```python
from build123d import *

# Parameters (mm, degrees)
SKETCH3_W = 15
SKETCH3_H = 18.520312213


with BuildPart() as part:
    # Sketch1 → Revolve1 (revolve)
    with BuildSketch(Plane.XY, mode=Mode.PRIVATE) as revolve1_sk:
        with BuildLine():
            Line((0, 41.73429327), (5, 41.73429327))
            Line((5, 41.73429327), (5, -108.26570673))
            ThreePointArc((5, -108.26570673), (9.659258263, -119.514151219), (0, -126.925960768))
            Line((0, -126.925960768), (0, 41.73429327))
        make_face()
    revolve(revolve1_sk.sketch.rotate(Axis((0, 41.73429327, 0), (0, -1, 0)), 180), axis=Axis((0, 41.73429327, 0), (0, -1, 0)))

    # Sketch3 → Revolve3 (revolve)
    with BuildSketch(Plane.XY, mode=Mode.PRIVATE) as revolve3_sk:
        with Locations((7.5, 32.474137164)):
            Rectangle(SKETCH3_W, SKETCH3_H)
    revolve(revolve3_sk.sketch.rotate(Axis((0, 41.73429327, 0), (0, -1, 0)), 90), axis=Axis((0, 41.73429327, 0), (0, -1, 0)))

    # Sketch5 → Cut-Revolve2 (revolve, cut)
    with BuildSketch(Plane.XY):
        with BuildLine():
            Line((0, 41.73429327), (0, 31.73429327))
            ThreePointArc((0, 31.73429327), (7.071067812, 34.663225458), (10, 41.73429327))
            Line((10, 41.73429327), (0, 41.73429327))
        make_face()
    revolve(axis=Axis((0, 41.73429327, 0), (0, -1, 0)), mode=Mode.SUBTRACT)


solid = part.part
```
Input: part model. Units: mm. Frame: model coordinates. Coordinates: 2 decimals unless noted, no trailing zeros. Loops run counter-clockwise (first coordinate to the right, second up) from the corner with the lowest first, then second, coordinate; pieces in that order, holes last.
Q1. Section A-A, the plane x = 6.5. Return the cut outline in (y, z).
Results are:
outline: circle Ø15.2 at (-116.93, 0); (23.21, -13.52) - (41.73, -13.52) - (41.73, -7.6) arc R7.6 cw to (41.73, 7.6) - (41.73, 13.52) - (23.21, 13.52) - close
Q2. Section B-B, the plane z = 0. Return the cut outline in (x, y).
Results are:
outline: (-15, 23.21) - (-5, 23.21) - (-5, -108.27) arc R10 ccw (long way) to (5, -108.27) - (5, 23.21) - (15, 23.21) - (15, 41.73) - (10, 41.73) arc R10 cw to (-10, 41.73) - (-15, 41.73) - close
Q3. Line query: line 1 along Y through (x, z) = (-3, 13.25); line 2 along Y through (x, z) = (3, -8.5); line 3 along Y through (x, z) = (6, -1). Output: solid intervals per line, ascending.
Results are:
line 1: y = 23.21 to 41.73
line 2: y = -121.26 to -112.6, 23.21 to 37.4
line 3: y = -124.86 to -108.99, 23.21 to 33.8
Q4. Contact query for flat-ended pins moving along their axis: pin 1 (5 mm diameter, centred on x = -7, y = 5, fed in from -Z); pin 2 (1 mm diameter, centred on x = -4, z = -1, fed in from -Y); pin 3 (8 mm diameter, centred on x = -8.5, y = -13, fed in from +Z). Output: stop coordinate, or through.
Results are:
pin 1: stops at z = -2.18
pin 2: stops at y = -126.25
pin 3: stops at z = 2.18
Q5. Section C-C, the plane x = 0. Return the cut outline in (y, z).
Results are:
outline: (-108.27, -5) - (23.21, -5) - (23.21, -15) - (41.73, -15) - (41.73, -10) arc R10 cw to (41.73, 10) - (41.73, 15) - (23.21, 15) - (23.21, 5) - (-108.27, 5) arc R10 ccw (long way) to start
Q6. Mould query, pull axis Y, two halves, no side actions, for faces 1 (the flat face through (10, 41.734, -3)), 2 (the cylindrical face through (-12.65, 32.6, 8.06)), 3 (the flat face through (-4, 23.214, 4)). Classes: +Y half, -Y half, draft (parallel to the pull), parting line (faces both ways), or undercut.
Results are:
face 1: +Y half
face 2: draft
face 3: undercut
Q7. Section D-D, the plane y = -72.5. Return the cut outline in (x, z).
Results are:
outline: circle Ø10 at (0, 0)
